Could you check a few things on this model? Use its own coordinates, in mm. Coordinates: 2 decimals unless noted, no trailing zeros. Order: outer loops, then holes, each group sorted by start corner. A loop starts at its lowest first (then second) coordinate and runs counter-clockwise, first axis right, second up. Notation, with made-up numbers: (19.5, -36) - (78.5, -36) arc R26 ccw to (78.5, -4) - close; hole circle Ø3 at (75.25, 45.5). An arc over 180 degrees is marked (long way). Answer as CSV lines item,"result". Start each with the question number.
1. I want a section at B-B, the plane y = -59. List the corners of the cut face in (x, z) for me.
2. I want a section at C-C, the plane y = -25. List the corners of the cut face in (x, z) for me, and give its area (3 significant figures).
3. I need wall thicknesses on probe 1 along Z at (x, y) = (6, -54); probe 2 along Z at (x, y) = (5.25, -35); probe 3 along Y at (x, z) = (1, -112.5). Which ranges of each line are inside material? Lowest first, please.
4. I want a section at A-A, the plane z = -93.5. List the corners of the cut face in (x, y) for me, and give its area (3 significant figures).
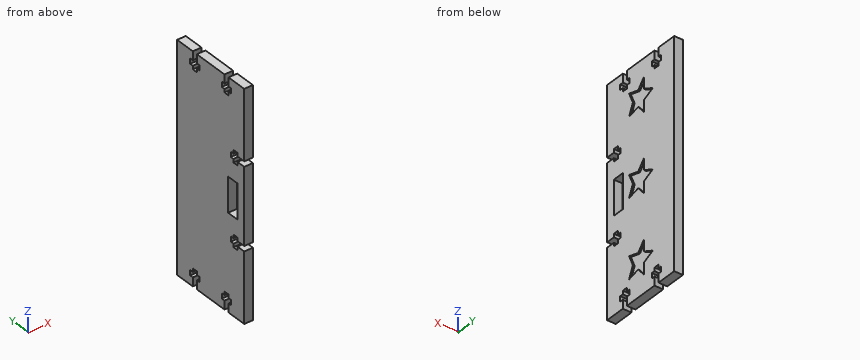
from build123d import *

# Parameters (mm, degrees)
BOSS_EXTRUDE1_DEPTH = 6.35
CUT_EXTRUDE1_DEPTH  = 178.004470283
CUT_EXTRUDE2_DEPTH  = 1.27
SKETCH4_W           = 25.4
SKETCH4_H           = 8.89
CUT_EXTRUDE3_DEPTH  = 178.004470283


with BuildPart() as part:
    # Sketch1 → Boss-Extrude1 (new body)
    with BuildSketch(Plane(origin=(0, 0, 0), x_dir=(0, 0, -1), z_dir=(1, 0, 0))):
        Polygon((0, 0), (165.1, 0), (165.1, -14.859), (158.75, -14.859), (158.75, -12.319), (154.94, -12.319), (154.94, -14.859), (152.4, -14.859), (152.4, -18.669), (154.94, -18.669), (154.94, -21.209), (158.75, -21.209), (158.75, -18.669), (165.1, -18.669), (165.1, -44.831), (158.75, -44.831), (158.75, -42.291), (154.94, -42.291), (154.94, -44.831), (152.4, -44.831), (152.4, -48.641), (154.94, -48.641), (154.94, -51.181), (158.75, -51.181), (158.75, -48.641), (165.1, -48.641), (165.1, -63.5), (0, -63.5), (0, -48.641), (6.35, -48.641), (6.35, -51.181), (10.16, -51.181), (10.16, -48.641), (12.7, -48.641), (12.7, -44.831), (10.16, -44.831), (10.16, -42.291), (6.35, -42.291), (6.35, -44.831), (0, -44.831), (0, -18.669), (6.35, -18.669), (6.35, -21.209), (10.16, -21.209), (10.16, -18.669), (12.7, -18.669), (12.7, -14.859), (10.16, -14.859), (10.16, -12.319), (6.35, -12.319), (6.35, -14.859), (0, -14.859), align=None)
    extrude(amount=BOSS_EXTRUDE1_DEPTH)

    # Sketch2 → Cut-Extrude1 (cut, through all)
    with BuildSketch(Plane(origin=(6.35, 0, 0), x_dir=(0, 0, -1), z_dir=(1, 0, 0))):
        Polygon((50.927, -63.5), (54.737, -63.5), (54.737, -57.15), (57.277, -57.15), (57.277, -53.34), (54.737, -53.34), (54.737, -50.8), (50.927, -50.8), (50.927, -53.34), (48.387, -53.34), (48.387, -57.15), (50.927, -57.15), align=None)
        Polygon((110.363, -63.5), (114.173, -63.5), (114.173, -57.15), (116.713, -57.15), (116.713, -53.34), (114.173, -53.34), (114.173, -50.8), (110.363, -50.8), (110.363, -53.34), (107.823, -53.34), (107.823, -57.15), (110.363, -57.15), align=None)
    extrude(amount=-CUT_EXTRUDE1_DEPTH, mode=Mode.SUBTRACT)

    # Sketch3 → Cut-Extrude2 (cut)
    with BuildSketch(Plane(origin=(6.35, 0, 0), x_dir=(0, 0, -1), z_dir=(1, 0, 0))):
        Polygon((82.55, -20.32), (78.792923653, -28.377076227), (69.902923653, -28.377076227), (76.713058752, -34.091458077), (74.412157441, -42.678538673), (82.55, -39.09976535), (90.687842559, -42.678538673), (88.386941248, -34.091458077), (95.197076347, -28.377076227), (86.307076347, -28.377076227), align=None)
        Polygon((25.4635, -20.32), (21.706423653, -28.377076227), (12.816423653, -28.377076227), (19.626558752, -34.091458077), (17.325657441, -42.678538673), (25.4635, -39.09976535), (33.601342559, -42.678538673), (31.300441248, -34.091458077), (38.110576347, -28.377076227), (29.220576347, -28.377076227), align=None)
        Polygon((139.6365, -20.32), (135.879423653, -28.377076227), (126.989423653, -28.377076227), (133.799558752, -34.091458077), (131.498657441, -42.678538673), (139.6365, -39.09976535), (147.774342559, -42.678538673), (145.473441248, -34.091458077), (152.283576347, -28.377076227), (143.393576347, -28.377076227), align=None)
    extrude(amount=-CUT_EXTRUDE2_DEPTH, mode=Mode.SUBTRACT)

    # Sketch4 → Cut-Extrude3 (cut, through all)
    with BuildSketch(Plane(origin=(6.35, 0, 0), x_dir=(0, 0, -1), z_dir=(1, 0, 0))):
        with Locations((82.55, -52.705)):
            Rectangle(SKETCH4_W, SKETCH4_H)
    extrude(amount=-CUT_EXTRUDE3_DEPTH, mode=Mode.SUBTRACT)


solid = part.part
Solved:
1,outline,"(0, -165.1) - (6.35, -165.1) - (6.35, -114.17) - (0, -114.17) - close; (0, -110.36) - (6.35, -110.36) - (6.35, -54.74) - (0, -54.74) - close; (0, -50.93) - (6.35, -50.93) - (6.35, 0) - (0, 0) - close"
2,outline,"(0, -165.1) - (6.35, -165.1) - (6.35, -141.82) - (5.08, -141.82) - (5.08, -137.45) - (6.35, -137.45) - (6.35, -84.73) - (5.08, -84.73) - (5.08, -80.37) - (6.35, -80.37) - (6.35, -27.65) - (5.08, -27.65) - (5.08, -23.28) - (6.35, -23.28) - (6.35, 0) - (0, 0) - close"
2,area,"1,030 mm2"
3,probe 1,"z = -165.1 to -116.71, -107.82 to -95.25, -69.85 to -57.28, -48.39 to 0"
3,probe 2,"z = -165.1 to -145.72, -133.56 to -88.63, -76.47 to -31.54, -19.38 to 0"
3,probe 3,"y = -50.8 to 0"
4,outline,"(0, -63.5) - (6.35, -63.5) - (6.35, -57.15) - (0, -57.15) - close; (0, -48.26) - (6.35, -48.26) - (6.35, -29.8) - (5.08, -29.8) - (5.08, -28.38) - (6.35, -28.38) - (6.35, 0) - (0, 0) - close"
4,area,"345 mm2"
